Verification items for the finished model (mm, model axes). A direction names the side the tool comes from. Give positions to 0.01 mm unless a question says otherwise; leave off trailing zeros. Loops run counter-clockwise (first coordinate to the right, second up) from the corner with the lowest first, then second, coordinate; pieces in that order, holes last. Notation, with made-up numbers: M 65.5,57 L 74.5,57 A31 ccw 74.5,95 Z; hole C 50,-31.5 d7. An arc over 180 degrees is marked long. Answer in a Markdown table with one row per item.
```python
from build123d import *

# Parameters (mm, degrees)
F1_R          = 12.5
F2_DEPTH      = 12
F4_DEPTH      = 25
F4_DEPTH_BACK = 25
F5_OFFSET     = 0.4


with BuildPart() as f2:
    # F1 (on Top) → F2 (new body)
    with BuildSketch(Plane.XY):
        Circle(F1_R)
    extrude(amount=F2_DEPTH)


with BuildPart() as f4:
    # F3 (on face) → F4 (new body, two sides)
    with BuildSketch(Plane.XY.offset(12)) as f4_sk:
        Polygon((0, -7.3323484187), (6.35, -3.6661742094), (6.35, 3.6661742094), (0, 7.3323484187), (-6.35, 3.6661742094), (-6.35, -3.6661742094), align=None)
    extrude(amount=-F4_DEPTH)
    extrude(f4_sk.sketch, amount=F4_DEPTH_BACK)


with BuildPart() as f2_1:
    add(f2.part)

    # F5: cut F4, made larger all round first
    f5_tool = offset(f4.part, amount=F5_OFFSET, kind=Kind.INTERSECTION, mode=Mode.PRIVATE)
    add(f5_tool, mode=Mode.SUBTRACT)


solid = f2_1.part
```
Item 1: Go/stop test with a flat-tipped pin: pin 1 (2 mm diameter, centred on x = 3.5, z = 9.5, fed in from +Y). Record where the tip stops, or that it passes through.
Reported:
| item | result |
|---|---|
| pin 1 | stops at y = 12.25 |
Item 2: Sectioned sample at A-A (y = 0). Record the cut outline in (x, z), and give its area (3 significant figures).
Reported:
| item | result |
|---|---|
| outline | M -12.5,0 L -6.75,0 L -6.75,12 L -12.5,12 Z; M 6.75,0 L 12.5,0 L 12.5,12 L 6.75,12 Z |
| area | 138 mm^2 |
Item 3: Scan lines: L1, parallel to Y at x = 1, z = 9.5; L2, parallel to Y at x = -0.25, z = 10.25; L3, parallel to X at y = 4, z = 5.5. Record each from-to range of solid material in increasing order. Write a range as [from, to].
Reported:
| item | result |
|---|---|
| L1 | y = [-12.46, -7.22], [7.22, 12.46] |
| L2 | y = [-12.5, -7.65], [7.65, 12.5] |
| L3 | x = [-11.84, -6.57], [6.57, 11.84] |
Item 4: Sectioned sample at D-D (y = 10). Record the cut outline in (x, z).
Reported:
| item | result |
|---|---|
| outline | M -7.5,0 L 7.5,0 L 7.5,12 L -7.5,12 Z |
Item 5: Release check for a two-part mould opening along X. For faces 1 (the cylindrical face through (11.923, 3.755, 5.916)), 2 (the flat face through (3.33, -5.87, 5.92)), 3 (the flat face through (5.4, -5.4, 0)) record: released by +X, released by -X, zero draft, split by the parting line, or undercut.
Reported:
| item | result |
|---|---|
| face 1 | split by the parting line |
| face 2 | undercut |
| face 3 | zero draft |
Item 6: Sectioned sample at B-B (z = 10.75). Record the cut outline in (x, y).
Reported:
| item | result |
|---|---|
| outline | C 0,0 d25; hole M -6.75,-3.9 L 0,-7.79 L 6.75,-3.9 L 6.75,3.9 L 0,7.79 L -6.75,3.9 Z |
Item 7: Tool access check on faces 4 (the flat face through (-6.75, 0, 6)), 5 (the flat face through (5.4, -5.4, 12)). Record the directions out of +Z, -Z, +X, -X, +Y, -Y that give a thin tool (end or side, any length) a straight path to the whole face; none if there is none.
Reported:
| item | result |
|---|---|
| face 4 | +Z, -Z |
| face 5 | +Z, +X, -X, +Y, -Y |
Item 8: Sectioned sample at C-C (x = -5). Record the cut outline in (y, z).
Reported:
| item | result |
|---|---|
| outline | M -11.46,0 L -4.91,0 L -4.91,12 L -11.46,12 Z; M 4.91,0 L 11.46,0 L 11.46,12 L 4.91,12 Z |
